from build123d import *

# Parameters (mm, degrees)
SKETCH2_W               = 1.651
SKETCH2_H               = 3.048
CUT_EXTRUDE1_DEPTH      = 10.525
CUT_EXTRUDE1_DEPTH_BACK = 10.525
CHAMFER1_SIZE           = 0.762


with BuildPart() as part:
    # Sketch1 → Revolve1 (revolve)
    with BuildSketch(Plane.XY):
        Polygon((-5.2451, -1.885785138), (-5.969, -10.16), (-8.001, -12.192), (-8.509, -12.192), (-8.509, -7.62), (-9.525, -6.604), (-9.525, 0.508), (-8.763, 1.27), (-5.2451, 1.27), (-5.2451, 0), align=None)
    revolve(axis=Axis((0, 0, 0), (0, -1, 0)))

    # Sketch2 → Cut-Extrude1 (cut, two sides)
    with BuildSketch(Plane.XY) as cut_extrude1_sk:
        with Locations((-8.6995, -0.254)):
            Rectangle(SKETCH2_W, SKETCH2_H)
        with Locations((8.6995, -0.254)):
            Rectangle(SKETCH2_W, SKETCH2_H)
    extrude(amount=CUT_EXTRUDE1_DEPTH, mode=Mode.SUBTRACT)
    extrude(cut_extrude1_sk.sketch, amount=-CUT_EXTRUDE1_DEPTH_BACK, mode=Mode.SUBTRACT)

    # Chamfer1
    chamfer1_edges = [part.edges().sort_by_distance(p)[0] for p in [
        (7.874, 1.27, 0),
        (-7.874, 1.27, 0),
    ]]
    chamfer(chamfer1_edges, length=CHAMFER1_SIZE)


solid = part.part
The listing builds one solid part. Answer for the finished solid, in the listing's coordinates (mm). A direction names the side the tool comes from. Give positions to 0.01 mm unless a question says otherwise; leave off trailing zeros. Write each loop counter-clockwise with the first axis right and the second up, starting at its lowest first coordinate (ties: lowest second). Pieces come first, ordered by that corner, then holes. Notation, with made-up numbers: (50, 19) - (100, 19) arc R11 cw to (100, 40) - close; hole circle Ø7 at (43.25, -32). An arc over 180 degrees is marked (long way). Use a Markdown table: item, result.
1. For a pull along X with two mould halves and no side action, classify faces 1 (the conical face through (0.72, -5.161, -5.485)), 2 (the conical face through (0.12, 1.15, 8.88)), 3 (the flat face through (-7.874, -1, 0)) as released by +X, released by -X, zero draft, split by the parting line, or undercut.
Values follow:
| item | result |
|---|---|
| face 1 | undercut |
| face 2 | split by the parting line |
| face 3 | released by -X |
2. Section A-A on z = 0 is taken. Write down the section's boundary in (x, y) (3 decimals), plus the area to 3 significant figures.
Values follow:
| item | result |
|---|---|
| outline | (-9.525, -6.604) - (-8.509, -7.62) - (-8.509, -12.192) - (-8.001, -12.192) - (-5.969, -10.16) - (-5.245, -1.886) - (-5.245, 1.27) - (-7.112, 1.27) - (-7.874, 0.508) - (-7.874, -1.778) - (-9.525, -1.778) - close; (5.245, -1.886) - (5.969, -10.16) - (8.001, -12.192) - (8.509, -12.192) - (8.509, -7.62) - (9.525, -6.604) - (9.525, -1.778) - (7.874, -1.778) - (7.874, 0.508) - (7.112, 1.27) - (5.245, 1.27) - close |
| area | 81.2 mm² |
3. Section D-D on y = -8.5 is taken. Write down the section's boundary in (x, z).
Values follow:
| item | result |
|---|---|
| outline | circle Ø17.02 at (0, 0); hole circle Ø11.65 at (0, 0) |
4. A tool of negligible diameter and unlimited length cuts with its end or side. For faces 4 (the flat face through (7.874, -1, 0)), 5 (the conical face through (-0.12, 1.15, -8.88)), 6 (the flat face through (-9, -1.778, 0)), 7 (the cylindrical face through (1.108, -9.874, -8.437)), 8 (the flat face through (0, 1.27, 6)), from which of +Z, -Z, +X, -X, +Y, -Y can it reach the whole face along a straight path? Write none if from no direction.
Values follow:
| item | result |
|---|---|
| face 4 | +Z, -Z, +X, +Y |
| face 5 | -Z, +Y |
| face 6 | +Z, -Z, -X, +Y |
| face 7 | -Y |
| face 8 | +Z, -Z, +X, -X, +Y |
5. Each of these flat-tipped pins is pushed along its axis until it touches: P1, Ø1.8, axis at y = 0, z = 0.5, coming from the +X side; P2, Ø1, axis at y = -8, z = -5, coming from the -X side; P3, Ø5, axis at y = -10, z = 4, coming from the +X side. Where does it stop, or does it pass through?
Values follow:
| item | result |
|---|---|
| P1 | stops at x = 7.87 |
| P2 | stops at x = -7.22 |
| P3 | stops at x = 8.38 |
6. Find the intervals of material crossed by probe 1 along X at (y, z) = (0.2, 0); probe 2 along Z at (x, y) = (0, -0.6) (3 decimals); probe 3 along Z at (x, y) = (3, -5.5), in increasing order. Write a range as from..to.
Values follow:
| item | result |
|---|---|
| probe 1 | x = -7.87..-5.25, 5.25..7.87 |
| probe 2 | z = -9.525..-5.245, 5.245..9.525 |
| probe 3 | z = -9.04..-4.68, 4.68..9.04 |
7. Section B-B on x = 0 is taken. Write down the section's boundary in (y, z) (3 decimals), plus the area to 3 significant figures.
Values follow:
| item | result |
|---|---|
| outline | (-12.192, -8.509) - (-7.62, -8.509) - (-6.604, -9.525) - (0.508, -9.525) - (1.27, -8.763) - (1.27, -5.245) - (-1.886, -5.245) - (-10.16, -5.969) - (-12.192, -8.001) - close; (-12.192, 8.001) - (-10.16, 5.969) - (-1.886, 5.245) - (1.27, 5.245) - (1.27, 8.763) - (0.508, 9.525) - (-6.604, 9.525) - (-7.62, 8.509) - (-12.192, 8.509) - close |
| area | 91.3 mm² |
8. Section C-C on y = -6 is taken. Write down the section's boundary in (x, z) (3 decimals), plus the area to 3 significant figures.
Values follow:
| item | result |
|---|---|
| outline | circle Ø19.05 at (0, 0); hole circle Ø11.21 at (0, 0) |
| area | 186 mm² |
